Geometry: final body of the model. Coordinates: model frame, mm. Face numbers are marked on the shaded views. A direction names the side the tool comes from. Give positions to 0.01 mm unless a question says otherwise; leave off trailing zeros. Loops run counter-clockwise (first coordinate to the right, second up) from the corner with the lowest first, then second, coordinate; pieces in that order, holes last.
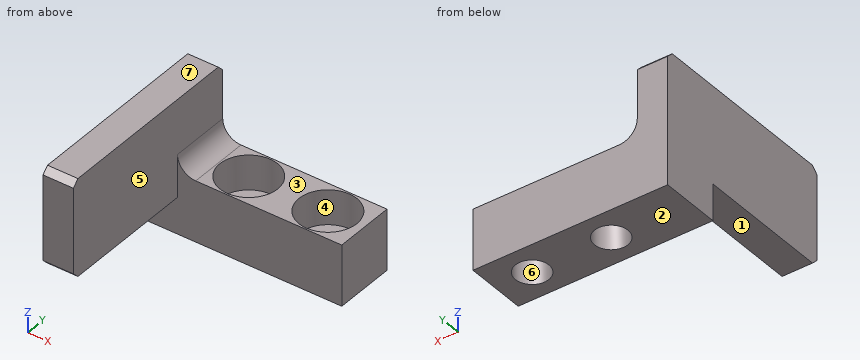
```python
from build123d import *

# Parameters (mm, degrees)
SKETCH_1_W                = 32
SKETCH_1_H                = 22
EXTRUDE_1_DEPTH           = 33
SKETCH_2_W                = 27
SKETCH_2_H                = 12
CUT_EXTRUDE_1_DEPTH       = 39.288379438
SKETCH_4_W                = 10
SKETCH_4_H                = 23
CUT_EXTRUDE_2_DEPTH       = 27
HOLE_WIZARD_1_D           = 5.5
HOLE_WIZARD_1_CBORE_D     = 9.5
HOLE_WIZARD_1_CBORE_DEPTH = 5.7
SKETCH_8_W                = 6
SKETCH_8_H                = 23
CUT_EXTRUDE_3_DEPTH       = 45.034077713
FILLET_1_R                = 3
CHAMFER_1_SIZE            = 1


with BuildPart() as part:
    # 草图1 → 凸台-拉伸1 (new body)
    with BuildSketch(Plane(origin=(0, 0, 0), x_dir=(1, 0, 0), z_dir=(0, 1, 0))):
        Rectangle(SKETCH_1_W, SKETCH_1_H)
    extrude(amount=EXTRUDE_1_DEPTH)

    # 草图2 → 切除-拉伸1 (cut, through all)
    with BuildSketch(Plane(origin=(0, 33, 0), x_dir=(1, 0, 0), z_dir=(0, 1, 0))):
        with Locations((2.5, -5)):
            Rectangle(SKETCH_2_W, SKETCH_2_H)
    extrude(amount=-CUT_EXTRUDE_1_DEPTH, mode=Mode.SUBTRACT)

    # 草图4 → 切除-拉伸2 (cut)
    with BuildSketch(Plane(origin=(16, 0, -21), x_dir=(0, 0, 1), z_dir=(-1, 0, 0))):
        with Locations((15, 11.5)):
            Rectangle(SKETCH_4_W, SKETCH_4_H)
    extrude(amount=CUT_EXTRUDE_2_DEPTH, mode=Mode.SUBTRACT)

    # 打孔尺寸根据内六角圆柱头螺钉的类型1 (through all)
    with Locations(Plane.XY.offset(-1)):
        with Locations((-3, 28), (10, 28)):
            CounterBoreHole(HOLE_WIZARD_1_D / 2, HOLE_WIZARD_1_CBORE_D / 2, HOLE_WIZARD_1_CBORE_DEPTH)

    # 草图8 → 切除-拉伸3 (cut, through all)
    with BuildSketch(Plane(origin=(-11, 0, 0), x_dir=(0, 0, -1), z_dir=(1, 0, 0))):
        with Locations((8, 11.5)):
            Rectangle(SKETCH_8_W, SKETCH_8_H)
    extrude(amount=-CUT_EXTRUDE_3_DEPTH, mode=Mode.SUBTRACT)

    # 圆角1
    fillet_1_edges = [part.edges().sort_by_distance(p)[0] for p in [
        (-11, 28, -1),
    ]]
    fillet(fillet_1_edges, radius=FILLET_1_R)

    # 倒角1
    chamfer_1_edges = [part.edges().sort_by_distance(p)[0] for p in [
        (-13.5, 33, 11),
        (-13.5, 0, 11),
        (-13.5, 0, -5),
    ]]
    chamfer(chamfer_1_edges, length=CHAMFER_1_SIZE)


solid = part.part
```
Q1. Section query D-D, the plane x = -4.5. Return loops of the section in (y, z).
Q2. Section query B-B, the plane y = 28. Return loops of the section in (x, z).
Q3. Mould query, pull axis X, two halves, no side actions, for the marked faces 5, 6 and 7. Classes: +X half, -X half, draft (parallel to the pull), parting line (faces both ways), or undercut.
Q4. Section query C-C, the plane z = -1.5. Return loops of the section in (x, y).
Q5. Reachability of the marked faces 1, 2, 3 and 4 from +Z, -Z, +X, -X, +Y, -Y: full face, straight path, thin tool, end or side. Return the list, or none.
Q6. Pin query (flat end, axial travel): pin 1 Ø4 at (x, y) = (-3.5, 22) entering from +Z; pin 2 Ø12 at (x, z) = (-2.5, 4.5) entering from -Y; pin 3 Ø12.5 at (x, y) = (-3, 28) entering from +Z. Return the tip coordinate at first contact, or that it passes through.
Q7. Material intervals for probe 1 along Y at (x, z) = (10, -3.95); probe 2 along X at (y, z) = (12, 4.75); probe 3 along Y at (x, z) = (7, -10), sorted ascending.
Q8. Section query A-A, the plane x = 10. Return loops of the section in (y, z).
Resolved:
1. outline: (23, -11) - (25.7, -11) - (25.7, -6.7) - (23.49, -6.7) - (23.49, -1) - (23, -1) - close; (30.3, -11) - (33, -11) - (33, -1) - (32.51, -1) - (32.51, -6.7) - (30.3, -6.7) - close
2. outline: (-16, -11) - (-5.75, -11) - (-5.75, -6.7) - (-7.75, -6.7) - (-7.75, -1) - (-8, -1) arc R3 cw to (-11, 2) - (-11, 11) - (-16, 11) - close; (-0.25, -11) - (7.25, -11) - (7.25, -6.7) - (5.25, -6.7) - (5.25, -1) - (1.75, -1) - (1.75, -6.7) - (-0.25, -6.7) - close; (12.75, -11) - (16, -11) - (16, -1) - (14.75, -1) - (14.75, -6.7) - (12.75, -6.7) - close
3. face 5: +X half
3. face 6: undercut
3. face 7: draft
4. outline: (-16, 0) - (-11, 0) - (-11, 23) - (16, 23) - (16, 33) - (-16, 33) - close; hole circle Ø9.5 at (-3, 28); hole circle Ø9.5 at (10, 28)
5. face 1: -Z, +X, -X, -Y
5. face 2: -Z, +X, -X, +Y, -Y
5. face 3: +Z, +X, +Y, -Y
5. face 4: +Z
6. pin 1: stops at z = -1
6. pin 2: stops at y = 23
6. pin 3: stops at z = -0.73
7. probe 1: y = 23 to 23.25, 32.75 to 33
7. probe 2: x = -16 to -11
7. probe 3: y = 23 to 33
8. outline: (23, -11) - (25.25, -11) - (25.25, -6.7) - (23.25, -6.7) - (23.25, -1) - (23, -1) - close; (30.75, -11) - (33, -11) - (33, -1) - (32.75, -1) - (32.75, -6.7) - (30.75, -6.7) - close
